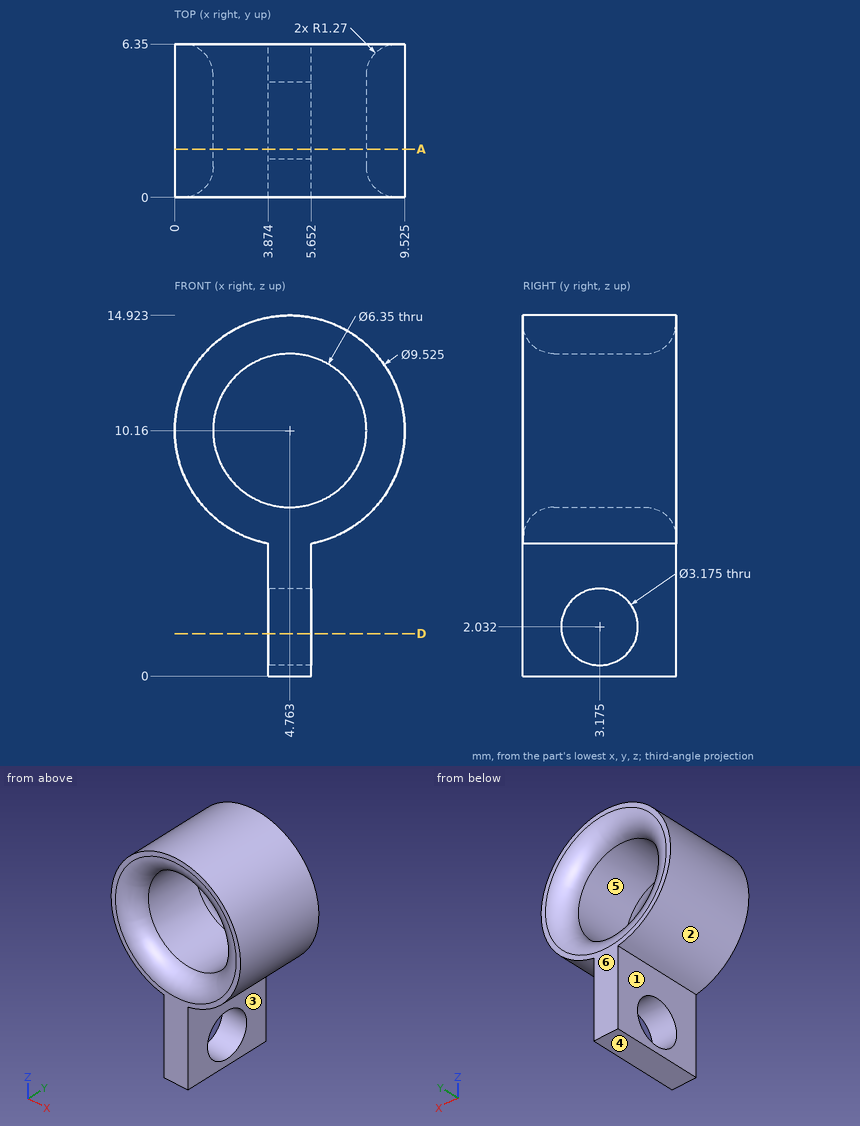
Drawing for the job (mm, zero at the part's lowest x, y, z). A direction names the side the tool comes from. Coordinates: 2 decimals unless noted, no trailing zeros. Order: outer loops, then holes, each group sorted by start corner. A loop starts at its lowest first (then second) coordinate and runs counter-clockwise, first axis right, second up.
Item 1: Band-saw the part on A-A on y = 2. Give the number of separate pieces and of enclosed holes in the cut face.
Check sheet entries:
separate pieces: 2
enclosed holes: 1
Item 2: Two-plate mould, pull along Z, no slides. Class the marked faces 4, 5 and 6: +Z half, -Z half, draft (parallel to the pull), parting line (faces both ways), or undercut.
Check sheet entries:
face 4: -Z half
face 5: undercut
face 6: draft
Item 3: Band-saw the part on D-D on z = 1.75. List the corners of the cut face in (x, y).
Check sheet entries:
outline: (3.87, 0) - (5.65, 0) - (5.65, 1.61) - (3.87, 1.61) - close; (3.87, 4.74) - (5.65, 4.74) - (5.65, 6.35) - (3.87, 6.35) - close
Item 4: Drill centre lines: L1, parallel to Z at x = 4.25, y = 2 (1 decimal); L2, parallel to X at y = 1.25, z = 10; L3, parallel to Z at x = 5.75, y = 4.75. Where is each one in solid material? Low to high.
Check sheet entries:
L1: z = 0 to 1, 3.1 to 7, 13.3 to 14.9
L2: x = 0 to 1.59, 7.93 to 9.52
L3: z = 5.5 to 7.14, 13.18 to 14.82
Item 5: 3-axis set-ups, long thin cutter, end or side, ignore diameter. For the marked faces 1, 2 and 3: which of +Z, -Z, +X, -X, +Y, -Y reach the whole face in a straight line?
Check sheet entries:
face 1: -Z, -X, +Y, -Y
face 2: +Y, -Y
face 3: -Z, +X, +Y, -Y
Item 6: Pin check, flat tips, straight feed: pin 1 Ø1.6 at (y, z) = (4.5, 2) entering from -X; pin 2 Ø3 at (y, z) = (4.5, 5.5) entering from +X (1 decimal); pin 3 Ø1.6 at (y, z) = (3, 4) entering from +X. Stop position of each tip, or through.
Check sheet entries:
pin 1: stops at x = 3.87
pin 2: stops at x = 8.3
pin 3: stops at x = 5.65
